Geometry: final body of the model. Coordinates: model frame, mm. A direction names the side the tool comes from. Give positions to 0.01 mm unless a question says otherwise; leave off trailing zeros. Order: outer loops, then holes, each group sorted by start corner. A loop starts at its lowest first (then second) coordinate and runs counter-clockwise, first axis right, second up. Notation, with made-up numbers: (43.25, -26) - (84.25, -26) arc R12 ccw to (84.25, -15) - close; hole circle Ø8 at (15, -4.75). An arc over 180 degrees is marked (long way). Use one line per item in the form item = value.
from build123d import *

# Parameters (mm, degrees)
F0_W     = 12
F0_H     = 3
F1_DEPTH = 10


with BuildPart() as f1:
    # F0 (on Right) → F1 (new body)
    with BuildSketch(Plane.YZ):
        Polygon((-15, 9), (-15, 0), (-12, 0), (-12, 6), (-12, 9), align=None)
        with Locations((-6, 7.5)):
            Rectangle(F0_W, F0_H)
        with Locations((6, 7.5)):
            Rectangle(F0_W, F0_H)
        Polygon((12, 9), (12, 6), (12, 0), (15, 0), (15, 9), align=None)
    extrude(amount=F1_DEPTH)


solid = f1.part
(1) Cut plane B-B on x = 5.5. Output: boundary loops of the cut face in (y, z), plus the area to 3 significant figures.
Computed values:
outline = (-15, 0) - (-12, 0) - (-12, 6) - (12, 6) - (12, 0) - (15, 0) - (15, 9) - (-15, 9) - close
area = 126 mm²
(2) Cut plane A-A on z = 1.75. Output: boundary loops of the cut face in (x, y).
Computed values:
outline = (0, -15) - (10, -15) - (10, -12) - (0, -12) - close; (0, 12) - (10, 12) - (10, 15) - (0, 15) - close
(3) Reachability of faces 1 (the face through (5, 0, 9)), 2 (the face through (5, -12, 3)) from +Z, -Z, +X, -X, +Y, -Y: full face, straight path, thin tool, end or side. Return the list, or none.
Computed values:
face_1 = +Z, +X, -X, +Y, -Y
face_2 = -Z, +X, -X
(4) Ray query, line 1 along Y through (x, z) = (4.75, 3.75); line 2 along Z through (x, y) = (6.75, -9.25). Return the intervals inside material, ascending.
Computed values:
line_1 = -15 to -12, 12 to 15
line_2 = 6 to 9
(5) Pull-direction query (Y, two-part tool) for faces 3 (the face through (5, 15, 4)), 4 (the face through (5, -14, 0)), 5 (the face through (5, 12, 3)); classes: released by +Y, released by -Y, zero draft, split by the parting line, or undercut.
Computed values:
face_3 = released by +Y
face_4 = zero draft
face_5 = undercut
(6) Cut plane C-C on y = -11.5. Output: boundary loops of the cut face in (x, z), plus the area to 3 significant figures.
Computed values:
outline = (0, 6) - (10, 6) - (10, 9) - (0, 9) - close
area = 30.0 mm²
